```python
from build123d import *

# Parameters (mm, degrees)
SKETCH2_W = 1.25
SKETCH2_H = 6
SKETCH4_W = 1.25
SKETCH4_H = 6


with BuildPart() as part:
    # Sketch1 → Revolve1 (revolve)
    with BuildSketch(Plane.XY):
        Polygon((0, 2.5), (0, 6), (6, 6), (6, 4.2291), (13, 4.2291), (13, 6), (14, 6), (14, 2.5), align=None)
    revolve(axis=Axis((0, 0, 0), (-1, 0, 0)))

    # Sketch2 → M3x0.5 Tapped Hole1 (revolve, cut)
    with BuildSketch(Plane(origin=(3, 0, 0), x_dir=(0, 0, -1), z_dir=(1, 0, 0))):
        with Locations((0.625, 3)):
            Rectangle(SKETCH2_W, SKETCH2_H)
    revolve(axis=Axis((3, -6.35, 0), (0, 1, 0)), mode=Mode.SUBTRACT)

    # Sketch4 → M3x0.5 Tapped Hole2 (revolve, cut)
    with BuildSketch(Plane.YZ.offset(3)):
        with Locations((0.625, 3)):
            Rectangle(SKETCH4_W, SKETCH4_H)
    revolve(axis=Axis((3, 0, -6.35), (0, 0, 1)), mode=Mode.SUBTRACT)


solid = part.part
```
The model under review builds one solid part; all positions refer to its coordinate system, in mm. A direction names the side the tool comes from. Give positions to 0.01 mm unless a question says otherwise; leave off trailing zeros. Loops run counter-clockwise (first coordinate to the right, second up) from the corner with the lowest first, then second, coordinate; pieces in that order, holes last. Notation, with made-up numbers: (-34, 70) -> (-29, 70) arc R25 ccw to (-29, 85) -> close; hole circle Ø1 at (78.5, 78). An arc over 180 degrees is marked (long way). Use CSV: the item, a comma, the result in double quotes.
1. The part is to be moulded in two halves that separate along Y. For faces 5 (the face through (6.9, -1.84, -1.69)), 6 (the face through (13.507, -5.994, -0.264)), 7 (the face through (0, -3, 0)), say which applies: +Y half, -Y half, draft (parallel to the pull), parting line (faces both ways), or undercut.
Result:
face 5,"undercut"
face 6,"parting line"
face 7,"draft"
2. For P1, Ø6, axis at x = 8, y = -3, coming from the -Z side; P2, Ø1.5, axis at x = 4, z = -3, coming from the +Y side; P3, Ø2, axis at x = 3, z = 0, coming from the +Y side, all flat-tipped, find the tip position at first contact; note any pin that passes through.
Result:
P1,"stops at z = -5.95"
P2,"stops at y = 5.56"
P3,"stops at y = -2.29"
3. Consider section C-C, the plane y = 5. Write out the cut boundary in (x, z).
Result:
outline,"(0, -3.32) -> (6, -3.32) -> (6, 3.32) -> (0, 3.32) -> close; (13, -3.32) -> (14, -3.32) -> (14, 3.32) -> (13, 3.32) -> close; hole circle Ø2.5 at (3, 0)"
4. To check wall thickness, follow probe 1 along X at (y, z) = (0, 5); probe 2 along X at (y, z) = (-4.5, 3.5); probe 3 along Z at (x, y) = (8, 0). State the ranges of each line that lie inside material, in increasing order. Write a range as from..to.
Result:
probe 1,"x = 0..1.75, 4.25..6, 13..14"
probe 2,"x = 0..6, 13..14"
probe 3,"z = -4.23..-2.5, 2.5..4.23"
5. Machinability: for faces 1 (the face through (2.95, -1.25, 4.11)), 2 (the face through (2.95, 4.11, 1.25)), 3 (the face through (9.549, -0.917, 4.129)), 4 (the face through (3, -6, 0)), which of the approach directions +Z, -Z, +X, -X, +Y, -Y give a long, thin tool a straight path to every point of the face, cutting with its end or side? Answer none if there is none.
Result:
face 1,"+Z"
face 2,"+Y"
face 3,"none"
face 4,"+X, -X"
6. Consider section A-A, the plane y = 0. Write out the cut boundary in (x, z), then the cut area to 3 significant figures.
Result:
outline,"(0, -6) -> (6, -6) -> (6, -4.23) -> (13, -4.23) -> (13, -6) -> (14, -6) -> (14, -2.5) -> (0, -2.5) -> close; (0, 2.5) -> (1.75, 2.5) -> (1.75, 6) -> (0, 6) -> close; (4.25, 2.5) -> (14, 2.5) -> (14, 6) -> (13, 6) -> (13, 4.23) -> (6, 4.23) -> (6, 6) -> (4.25, 6) -> close"
area,"64.5 mm²"
7. Consider section D-D, the plane x = 6.25. Write out the cut boundary in (y, z).
Result:
outline,"circle Ø8.46 at (0, 0); hole circle Ø5 at (0, 0)"
